Build history of the part. All positions in model axes, mm. Round coordinates to 2 decimals unless told otherwise and drop trailing zeros. Loops run counter-clockwise (first coordinate to the right, second up) from the corner with the lowest first, then second, coordinate; pieces in that order, holes last. Notation, with made-up numbers: (-24.5, 6.5) - (6.5, 6.5) arc R12 cw to (6.5, 20.5) - close; hole circle Ø2 at (-35.75, -24). An arc over 180 degrees is marked (long way). Use one line per item in the form item = value. Start each with the question number.
Q1. Saw through at A-A (x = 0). Give the cut face in (y, z) (3 decimals).
Q2. Pin check, flat tips, straight feed: pin 1 (8 mm diameter, centred on x = 1.5, z = 10, fed in from -Y); pin 2 (1 mm diameter, centred on y = -5.5, z = -20, fed in from -X). Stop position of each tip, or through.
Q3. Saw through at B-B (z = 0). Give the cut face in (x, y), then the cut area to 3 significant figures.
Q4. Saw through at D-D (y = -3.5). Count the separate pieces of the cut face and the enclosed holes in it, then the cut area to 3 significant figures.
Q5. Drill centre lines: line 1 (Z direction, x = -32, y = -5.5) (3 decimals); line 2 (Z direction, x = 0, y = -2) (3 decimals); line 3 (X direction, y = -4.5, z = 7). Where is each one in solid material? Low to high.
Q6. Saw through at C-C (z = 11). Give the cut face in (x, y), then the cut area to 3 significant figures.
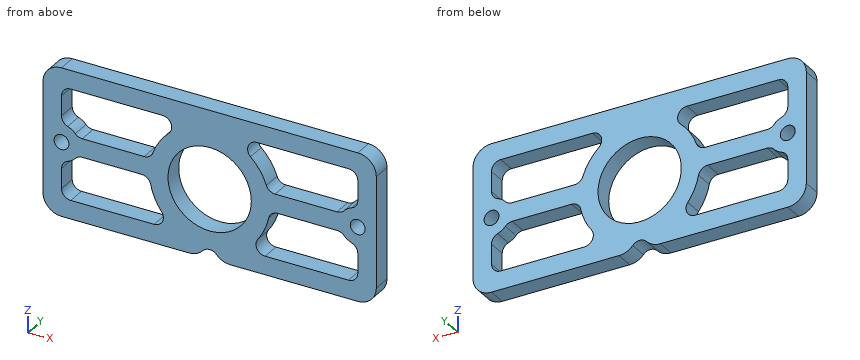
```python
from build123d import *

# Parameters (mm, degrees)
F0_R     = 14.2875
F0_R_2   = 2.5527
F1_DEPTH = 6.35
F2_R     = 6.35
F4_DEPTH = 25.4


with BuildPart() as f1:
    # F0 (on Front) → F1 (new body)
    with BuildSketch(Plane.XZ):
        with BuildLine():
            Line((57.15, 25.4), (-57.15, 25.4))
            Line((-57.15, 25.4), (-57.15, -25.4))
            Line((-57.15, -25.4), (-3.175, -25.4))
            ThreePointArc((-3.175, -25.4), (0, -22.225), (3.175, -25.4))
            Line((3.175, -25.4), (57.15, -25.4))
            Line((57.15, -25.4), (57.15, 25.4))
        make_face()
        with Locations((0, -1.5875)):
            Circle(F0_R, mode=Mode.SUBTRACT)
        with Locations((-50.8, 0)):
            Circle(F0_R_2, mode=Mode.SUBTRACT)
        with Locations((50.8, 0)):
            Circle(F0_R_2, mode=Mode.SUBTRACT)
    extrude(amount=F1_DEPTH)

    # F2
    f2_edges = [f1.edges().sort_by_distance(p)[0] for p in [
        (-57.15, -3.175, 25.4),
        (-57.15, -3.175, -25.4),
        (57.15, -3.175, -25.4),
        (57.15, -3.175, 25.4),
        (-3.175, -3.175, -25.4),
        (3.175, -3.175, -25.4),
    ]]
    fillet(f2_edges, radius=F2_R)

    # F3 (on face) → F4 (cut)
    with BuildSketch(Plane.XZ.offset(6.35)):
        with BuildLine():
            ThreePointArc((-46.066989, 4.233333), (-44.996672, 3.451635), (-43.700484, 3.175))
            Line((-43.700484, 3.175), (-22.45064, 3.175))
            ThreePointArc((-22.45064, 3.175), (-20.617553, 3.757623), (-19.457222, 5.291667))
            ThreePointArc((-19.457222, 5.291667), (-17.245237, 9.748647), (-14.030802, 13.546667))
            ThreePointArc((-14.030802, 13.546667), (-13.233623, 17.034346), (-16.189387, 19.05))
            Line((-16.189387, 19.05), (-47.625, 19.05))
            ThreePointArc((-47.625, 19.05), (-49.870064, 18.120064), (-50.8, 15.875))
            Line((-50.8, 15.875), (-50.8, 8.980256))
            ThreePointArc((-50.8, 8.980256), (-50.217377, 7.147169), (-48.683333, 5.986837))
            ThreePointArc((-48.683333, 5.986837), (-47.264719, 5.274873), (-46.066989, 4.233333))
        make_face()
        with BuildLine():
            Line((-23.33139, -3.175), (-43.700484, -3.175))
            ThreePointArc((-43.700484, -3.175), (-44.996672, -3.451635), (-46.066989, -4.233333))
            ThreePointArc((-46.066989, -4.233333), (-47.264719, -5.274873), (-48.683333, -5.986837))
            ThreePointArc((-48.683333, -5.986837), (-50.217377, -7.147169), (-50.8, -8.980256))
            Line((-50.8, -8.980256), (-50.8, -15.875))
            ThreePointArc((-50.8, -15.875), (-49.870064, -18.120064), (-47.625, -19.05))
            Line((-47.625, -19.05), (-19.05, -19.05))
            ThreePointArc((-19.05, -19.05), (-16.210194, -17.294903), (-16.51, -13.97))
            ThreePointArc((-16.51, -13.97), (-18.823373, -10.048413), (-20.220538, -5.715))
            ThreePointArc((-20.220538, -5.715), (-21.323343, -3.890656), (-23.33139, -3.175))
        make_face()
        with BuildLine():
            ThreePointArc((43.700484, 3.175), (44.996672, 3.451635), (46.066989, 4.233333))
            ThreePointArc((46.066989, 4.233333), (47.264719, 5.274873), (48.683333, 5.986837))
            ThreePointArc((48.683333, 5.986837), (50.217377, 7.147169), (50.8, 8.980256))
            Line((50.8, 8.980256), (50.8, 15.875))
            ThreePointArc((50.8, 15.875), (49.870064, 18.120064), (47.625, 19.05))
            Line((47.625, 19.05), (16.189387, 19.05))
            ThreePointArc((16.189387, 19.05), (13.233623, 17.034346), (14.030802, 13.546667))
            ThreePointArc((14.030802, 13.546667), (17.245237, 9.748647), (19.457222, 5.291667))
            ThreePointArc((19.457222, 5.291667), (20.617553, 3.757623), (22.45064, 3.175))
            Line((22.45064, 3.175), (43.700484, 3.175))
        make_face()
        with BuildLine():
            ThreePointArc((50.8, -8.980256), (50.217377, -7.147169), (48.683333, -5.986837))
            ThreePointArc((48.683333, -5.986837), (47.264719, -5.274873), (46.066989, -4.233333))
            ThreePointArc((46.066989, -4.233333), (44.996672, -3.451635), (43.700484, -3.175))
            Line((43.700484, -3.175), (23.33139, -3.175))
            ThreePointArc((23.33139, -3.175), (21.323343, -3.890656), (20.220538, -5.715))
            ThreePointArc((20.220538, -5.715), (18.823373, -10.048413), (16.51, -13.97))
            ThreePointArc((16.51, -13.97), (16.210194, -17.294903), (19.05, -19.05))
            Line((19.05, -19.05), (47.625, -19.05))
            ThreePointArc((47.625, -19.05), (49.870064, -18.120064), (50.8, -15.875))
            Line((50.8, -15.875), (50.8, -8.980256))
        make_face()
    extrude(amount=-F4_DEPTH, mode=Mode.SUBTRACT)


solid = f1.part
```
Report:
q1.outline = (-6.35, -22.225) - (0, -22.225) - (0, -15.875) - (-6.35, -15.875) - close; (-6.35, 12.7) - (0, 12.7) - (0, 25.4) - (-6.35, 25.4) - close
q2.pin_1 = -6.35
q2.pin_2 = -57.13
q3.outline = (-57.15, -6.35) - (-53.35, -6.35) - (-53.35, 0) - (-57.15, 0) - close; (-48.25, -6.35) - (-14.2, -6.35) - (-14.2, 0) - (-48.25, 0) - close; (14.2, -6.35) - (48.25, -6.35) - (48.25, 0) - (14.2, 0) - close; (53.35, -6.35) - (57.15, -6.35) - (57.15, 0) - (53.35, 0) - close
q3.area = 481 mm²
q4.separate_pieces = 1
q4.enclosed_holes = 7
q4.area = 3,010 mm²
q5.line_1 = -25.4 to -19.05, -3.175 to 3.175, 19.05 to 25.4
q5.line_2 = -22.225 to -15.875, 12.7 to 25.4
q5.line_3 = -57.15 to -50.11, -18.77 to -11.42, 11.42 to 18.77, 50.11 to 57.15
q6.outline = (-57.15, -6.35) - (-50.8, -6.35) - (-50.8, 0) - (-57.15, 0) - close; (-16.35, -6.35) - (-6.76, -6.35) - (-6.76, 0) - (-16.35, 0) - close; (6.76, -6.35) - (16.35, -6.35) - (16.35, 0) - (6.76, 0) - close; (50.8, -6.35) - (57.15, -6.35) - (57.15, 0) - (50.8, 0) - close
q6.area = 203 mm²
